CAD build for the part. Positions are in the model's coordinates, mm. A direction names the side the tool comes from. Give positions to 0.01 mm unless a question says otherwise; leave off trailing zeros. Write each loop counter-clockwise with the first axis right and the second up, starting at its lowest first coordinate (ties: lowest second). Pieces come first, ordered by that corner, then holes. Notation, with made-up numbers: (-37.5, 31.25) - (18.5, 31.25) arc R17 ccw to (18.5, 51.25) - close; hole circle Ø5 at (86.5, 71). An arc over 180 degrees is marked (long way). Answer as a JSON object with one key per item and string values.
from build123d import *

# Parameters (mm, degrees)
ESQUISSE1_W                                = 48.3
ESQUISSE1_H                                = 42.3
ESQUISSE1_R                                = 11.5
ESQUISSE1_R_2                              = 1.65
BOSS_EXTRU_1_DEPTH                         = 4
ESQUISSE2_W                                = 48.3
ESQUISSE2_H                                = 51
BOSS_EXTRU_2_DEPTH                         = 3
BOSS_EXTRU_3_DEPTH                         = 3
CONG_1_R                                   = 10
CHANFREIN1_SIZE                            = 0.5
CHANFREIN2_SIZE                            = 0.5
FRAISAGE_POUR_VIS_T_TE_FRAIS_E_BOM_2_COUNT = 2
FRAISAGE_POUR_VIS_T_TE_FRAIS_E_BOM_2_PITCH = 30.528675045
FRAISAGE_POUR_VIS_T_TE_FRAIS_E_BOM_3_COUNT = 2
FRAISAGE_POUR_VIS_T_TE_FRAIS_E_BOM_3_PITCH = 30.528675045


with BuildPart() as part:
    # Esquisse1 → Boss.-Extru.1 (new body)
    with BuildSketch(Plane.XY):
        Rectangle(ESQUISSE1_W, ESQUISSE1_H)
        Circle(ESQUISSE1_R, mode=Mode.SUBTRACT)
        with Locations((-15.5, 15.5)):
            Circle(ESQUISSE1_R_2, mode=Mode.SUBTRACT)
        with Locations((15.5, 15.5)):
            Circle(ESQUISSE1_R_2, mode=Mode.SUBTRACT)
        with Locations((15.5, -15.5)):
            Circle(ESQUISSE1_R_2, mode=Mode.SUBTRACT)
        with Locations((-15.5, -15.5)):
            Circle(ESQUISSE1_R_2, mode=Mode.SUBTRACT)
    extrude(amount=BOSS_EXTRU_1_DEPTH)

    # Esquisse2 → Boss.-Extru.2 (add)
    with BuildSketch(Plane.XZ.offset(21.15)):
        with Locations((0, -21.5)):
            Rectangle(ESQUISSE2_W, ESQUISSE2_H)
    extrude(amount=BOSS_EXTRU_2_DEPTH)

    # Esquisse3 → Boss.-Extru.3 (add)
    with BuildSketch(Plane.ZY.offset(24.15)):
        Polygon((0, 3.85), (-25, -21.15), (0, -21.15), align=None)
    boss_extru_3 = extrude(amount=-BOSS_EXTRU_3_DEPTH)

    # Symétrie1: Boss.-Extru.3 across plane
    add(boss_extru_3.mirror(Plane(origin=(0, 0, 0), x_dir=(0, 0, 1), z_dir=(1, 0, 0))))

    # Congé1
    cong_1_edges = [part.edges().sort_by_distance(p)[0] for p in [
        (-22.65, 3.85, 0),
        (-22.65, -21.15, -25),
        (22.65, 3.85, 0),
        (22.65, -21.15, -25),
    ]]
    fillet(cong_1_edges, radius=CONG_1_R)

    # Chanfrein1
    chanfrein1_edges = [part.edges().sort_by_distance(p)[0] for p in [
        (-11.5, 0, 4),
        (24.15, -1.5, 4),
        (-17.15, 15.5, 4),
        (0, 21.15, 4),
        (13.85, 15.5, 4),
        (13.85, -15.5, 4),
        (-17.15, -15.5, 4),
        (0, -24.15, 4),
        (-24.15, -1.5, 4),
    ]]
    chamfer(chanfrein1_edges, length=CHANFREIN1_SIZE)

    # Chanfrein2
    chanfrein2_edges = [part.edges().sort_by_distance(p)[0] for p in [
        (-11.5, 0, 0),
    ]]
    chamfer(chanfrein2_edges, length=CHANFREIN2_SIZE)

    # Esquisse4 → Fraisage pour vis à tête fraisée bombée fendue M51 (revolve, cut)
    with BuildSketch(Plane(origin=(0, -21.15, -11), x_dir=(0, 0, 1), z_dir=(1, 0, 0))):
        Polygon((0, 0), (0, 3), (2.75, 3), (2.75, 2.85), (5.6, 0), align=None)
    fraisage_pour_vis_t_te_frais_e_bomb_e = revolve(axis=Axis((0, -14.8, -11), (0, -1, 0)), mode=Mode.SUBTRACT)

    # Fraisage pour vis _ t_te frais_e bom 2: Fraisage pour vis à tête fraisée bombée fendue M51 ×2
    with Locations(*[Vector(0.5240974256643348, 0, -0.8516583167045438) * (i * FRAISAGE_POUR_VIS_T_TE_FRAIS_E_BOM_2_PITCH) for i in range(1, FRAISAGE_POUR_VIS_T_TE_FRAIS_E_BOM_2_COUNT)]):
        add(fraisage_pour_vis_t_te_frais_e_bomb_e, mode=Mode.SUBTRACT)

    # Fraisage pour vis _ t_te frais_e bom 3: Fraisage pour vis à tête fraisée bombée fendue M51 ×2
    with Locations(*[Vector(-0.5240974256643347, 0, -0.851658316704544) * (i * FRAISAGE_POUR_VIS_T_TE_FRAIS_E_BOM_3_PITCH) for i in range(1, FRAISAGE_POUR_VIS_T_TE_FRAIS_E_BOM_3_COUNT)]):
        add(fraisage_pour_vis_t_te_frais_e_bomb_e, mode=Mode.SUBTRACT)


solid = part.part
Item 1: Cut at B-B (x = 0). Give the cut face in (y, z).
Entries:
{"outline": "(-24.15, -47) - (-21.15, -47) - (-21.15, -16.6) - (-24, -13.75) - (-24.15, -13.75) - close; (-24.15, -8.25) - (-24, -8.25) - (-21.15, -5.4) - (-21.15, 0) - (-12, 0) - (-11.5, 0.5) - (-11.5, 3.5) - (-12, 4) - (-23.65, 4) - (-24.15, 3.5) - close; (11.5, 0.5) - (12, 0) - (21.15, 0) - (21.15, 3.5) - (20.65, 4) - (12, 4) - (11.5, 3.5) - close"}
Item 2: Cut at D-D (y = 0). Give the cut face in (x, z), and give its area (3 significant figures).
Entries:
{"outline": "(-24.15, -3.85) - (-21.15, -3.85) - (-21.15, 0) - (-12, 0) - (-11.5, 0.5) - (-11.5, 3.5) - (-12, 4) - (-23.65, 4) - (-24.15, 3.5) - close; (11.5, 0.5) - (12, 0) - (21.15, 0) - (21.15, -3.85) - (24.15, -3.85) - (24.15, 3.5) - (23.65, 4) - (12, 4) - (11.5, 3.5) - close", "area": "124 mm2"}
Item 3: Which spindle directions (+Z, -Z, +X, -X, +Y, -Y) get a long thin tool onto all of the face, cutting with end or side? Do faces 3 (the cylindrical face through (22.629, 4.115, -0.782)), 4 (the flat face through (21.15, -14, -8)). Say none if no direction does.
Entries:
{"face 3": "-Z, +X, -X, +Y", "face 4": "-Z, +Y"}
Item 4: Cut at A-A (y = -15.5). Give the cut face in (x, z), and give its area (3 significant figures).
Entries:
{"outline": "(-24.15, -19.35) - (-21.15, -19.35) - (-21.15, 0) - (-17.15, 0) - (-17.15, 3.5) - (-17.65, 4) - (-23.65, 4) - (-24.15, 3.5) - close; (-13.85, 0) - (13.85, 0) - (13.85, 3.5) - (13.35, 4) - (-13.35, 4) - (-13.85, 3.5) - close; (17.15, 0) - (21.15, 0) - (21.15, -19.35) - (24.15, -19.35) - (24.15, 3.5) - (23.65, 4) - (17.65, 4) - (17.15, 3.5) - close", "area": "282 mm2"}
Item 5: Flat gauge pins, fed straight in: P1, Ø4.5, axis at x = -15.5, y = 15.5, coming from the +Z side; P2, Ø3, axis at x = 2.5, z = -25, coming from the +Y side; P3, Ø7, axis at x = 0, z = -11, coming from the +Y side; P4, Ø12.5, axis at x = -8, y = -4.5, coming from the -Z side. Where does each tip first touch, or does it go through?
Entries:
{"P1": "z = 4", "P2": "y = -21.15", "P3": "y = -23.25", "P4": "z = 0"}
Item 6: Probe line 1 (Y direction, x = -15.5, z = 0.75); line 2 (X direction, y = -24.05, z = -37); line 3 (Y direction, x = 0, z = 1). List the from-to ranges inside material, lowest first. Write a range as from..to.
Entries:
{"line 1": "-24.15..-17.15, -13.85..13.85, 17.15..21.15", "line 2": "-24.15..-18.75, -13.25..13.25, 18.75..24.15", "line 3": "-24.15..-11.5, 11.5..21.15"}
Item 7: Mould opens along X. For faces 1 (the flat face through (0, -23, -47)), 2 (the cylindrical face through (-13.926, -15.004, 1.726)) say: +X half, -X half, draft (parallel to the pull), parting line (faces both ways), or undercut.
Entries:
{"face 1": "draft", "face 2": "undercut"}
Item 8: Cut at C-C (z = -11). Give the cut face in (x, y), and give its area (3 significant figures).
Entries:
{"outline": "(-24.15, -24.15) - (-2.75, -24.15) - (-2.75, -24) - (-5.6, -21.15) - (-21.15, -21.15) - (-21.15, -7.15) - (-24.15, -7.15) - close; (2.75, -24.15) - (24.15, -24.15) - (24.15, -7.15) - (21.15, -7.15) - (21.15, -21.15) - (5.6, -21.15) - (2.75, -24) - close", "area": "204 mm2"}
